```python
from build123d import *

# Parameters (mm, degrees)
SKETCH_1_R          = 58
EXTRUDE_1_DEPTH     = 8
FILLET_1_R          = 10
FILLET_2_R          = 10
SKETCH_6_R          = 1.7526
CUT_EXTRUDE_1_DEPTH = 20


with BuildPart() as part:
    # 草图1 → 凸台-拉伸1 (new body)
    with BuildSketch(Plane(origin=(0, 0, 0), x_dir=(1, 0, 0), z_dir=(0, 1, 0))):
        with Locations(Location((0, 0, 0), (0, 0, 270))):
            Circle(SKETCH_1_R)
        with BuildLine():
            Line((-5, 53.768020235), (-5, 8.660254038))
            ThreePointArc((-5, 8.660254038), (-7.071067812, 7.071067812), (-8.660254038, 5))
            Line((-8.660254038, 5), (-53.768020235, 5))
            ThreePointArc((-53.768020235, 5), (-38.183766184, 38.183766184), (-5, 53.768020235))
        make_face(mode=Mode.SUBTRACT)
        with BuildLine():
            Line((-53.768020235, -5), (-8.660254038, -5))
            ThreePointArc((-8.660254038, -5), (-7.071067812, -7.071067812), (-5, -8.660254038))
            Line((-5, -8.660254038), (-5, -53.768020235))
            ThreePointArc((-5, -53.768020235), (-38.183766184, -38.183766184), (-53.768020235, -5))
        make_face(mode=Mode.SUBTRACT)
        with BuildLine():
            Line((5, -53.768020235), (5, -8.660254038))
            ThreePointArc((5, -8.660254038), (7.071067812, -7.071067812), (8.660254038, -5))
            Line((8.660254038, -5), (53.768020235, -5))
            ThreePointArc((53.768020235, -5), (38.183766184, -38.183766184), (5, -53.768020235))
        make_face(mode=Mode.SUBTRACT)
        with BuildLine():
            Line((53.768020235, 5), (8.660254038, 5))
            ThreePointArc((8.660254038, 5), (7.071067812, 7.071067812), (5, 8.660254038))
            Line((5, 8.660254038), (5, 53.768020235))
            ThreePointArc((5, 53.768020235), (38.183766184, 38.183766184), (53.768020235, 5))
        make_face(mode=Mode.SUBTRACT)
    extrude(amount=EXTRUDE_1_DEPTH)

    # 圆角1
    fillet_1_edges = [part.edges().sort_by_distance(p)[0] for p in [
        (53.768020235, 4, 5),
        (5, 4, 53.768020235),
        (53.768020235, 4, -5),
        (5, 4, -53.768020235),
        (-5, 4, -53.768020235),
        (-53.768020235, 4, -5),
        (-53.768020235, 4, 5),
        (-5, 4, 53.768020235),
    ]]
    fillet(fillet_1_edges, radius=FILLET_1_R)

    # 圆角2
    # the kernel refuses this fillet: 10 mm, written as the material it adds along each edge
    with BuildSketch(Plane(origin=(5, 0, -8.660254038), x_dir=(0, 0, -1), z_dir=(0, 1, 0)), Plane(origin=(-5, 0, 8.660254038), x_dir=(0, 0, 1), z_dir=(0, 1, 0)), Plane(origin=(-8.660254038, 0, -5), x_dir=(-1, 0, 0), z_dir=(0, 1, 0))) as fillet_2_piece_1:
        with BuildLine():
            CenterArc((4.568502517, -10), FILLET_2_R, 90, 41.409622109)
            ThreePointArc((-2.04587576, -2.5), (-0.921320126, -1.33315892), (0, 0))
            Line((0, 0), (4.568502517, 0))
        make_face()
    extrude(amount=8)
    with BuildSketch(Plane(origin=(8.660254038, 0, -5), x_dir=(1, 0, 0), z_dir=(0, 1, 0)), Plane(origin=(5, 0, 8.660254038), x_dir=(0, 0, 1), z_dir=(0, 1, 0)), Plane(origin=(-8.660254038, 0, 5), x_dir=(-1, 0, 0), z_dir=(0, 1, 0)), Plane(origin=(-5, 0, -8.660254038), x_dir=(0, 0, -1), z_dir=(0, 1, 0))) as fillet_2_piece_2:
        with BuildLine():
            CenterArc((4.568502517, 10), FILLET_2_R, 228.590377891, 41.409622109)
            ThreePointArc((-2.04587576, 2.5), (-0.921320126, 1.33315892), (0, 0))
            Line((0, 0), (4.568502517, 0))
        make_face()
    extrude(amount=8)
    with BuildSketch(Plane(origin=(8.660254038, 0, 5), x_dir=(-0.6333158920043416, 0, 0.7738933911946432), z_dir=(0, 1, 0))) as fillet_2_piece_3:
        with BuildLine():
            CenterArc((4.845628665, 9.868692826), FILLET_2_R, 219.295188945, 41.409622109)
            Line((-2.893305247, 3.535533906), (0, 0))
            ThreePointArc((0, 0), (1.615209555, 0.131307174), (3.23041911, 0))
        make_face()
    extrude(amount=8)

    # 切除-扫描1: sweep along a path in 草图5
    with BuildLine(Plane(origin=(0, 4, 0), x_dir=(1, 0, 0), z_dir=(0, 1, 0))) as sweep_1_path:
        CenterArc((0, 0), 58, 0, 360)
    # 草图6 → 切除-扫描1 (sweep, cut)
    with BuildSketch(Plane.XY):
        with Locations((-58, 4)):
            Circle(SKETCH_6_R)
    sweep(path=sweep_1_path.line, mode=Mode.SUBTRACT)

    # 草图7 → 切除-拉伸1 (cut)
    with BuildSketch(Plane(origin=(0, 0, 0), x_dir=(-1, 0, 0), z_dir=(0, -1, 0))):
        with BuildLine():
            Line((-1.118033989, -1), (-0.213422781, -1))
            Line((-0.213422781, -1), (1.118033989, -1))
            ThreePointArc((1.118033989, -1), (1.401258538, -0.535233135), (1.5, 0))
            ThreePointArc((1.5, 0), (-0.535233135, 1.401258538), (-1.118033989, -1))
        make_face()
    extrude(amount=-CUT_EXTRUDE_1_DEPTH, mode=Mode.SUBTRACT)


solid = part.part
```
Geometry: final body of the model. Coordinates: model frame, mm. Coordinates: 2 decimals unless noted, no trailing zeros. Use CSV: the item, a comma, the result in double quotes. Start each with the question number.
1. Ray query, probe 1 along Z at (x, y) = (0, 6); probe 2 along Z at (x, y) = (7, 4.5); probe 3 along X at (y, z) = (5, -35). Return the intervals inside material, ascending.
2. Cut plane A-A on x = -11.5. Count the separate pieces of the cut face and the enclosed holes in it, plus the area to 3 significant figures.
3. First-contact query: P1, Ø2, axis at x = -27.5, y = 4.5, coming from the +Z side; P2, Ø4, axis at x = 26.5, y = 3, coming from the -Z side; P3, Ø3, axis at x = -22.5, y = 1.5, coming from the +Z side. Flat tips, straight axial feed; report the tip coordinate or a pass-through.
Entries:
1,probe 1,"-58 to -1.5, 1 to 58"
1,probe 2,"-55.88 to -47.36, -7.23 to 7.23, 47.36 to 55.88"
1,probe 3,"-44.43 to -41.12, -5 to 5, 41.12 to 44.43"
2,separate pieces,"3"
2,enclosed holes,"0"
2,area,"170 mm²"
3,P1,"z = 50.12"
3,P2,"z = -52.5"
3,P3,"z = 54.06"
